```python
from build123d import *

# Parameters (mm, degrees)
BOSS_EXTRUDE1_DEPTH  = 10
CHAMFER1_SIZE        = 5
CHAMFER2_SIZE        = 2
CHAMFER3_SIZE        = 1
CUT_EXTRUDE1_DEPTH   = 3
M3_CLEARANCE_HOLE1_D = 3.4
CUT_EXTRUDE2_DEPTH   = 3


with BuildPart() as part:
    # Sketch1 → Boss-Extrude1 (new body)
    with BuildSketch(Plane(origin=(0, 0, 0), x_dir=(1, 0, 0), z_dir=(0, 1, 0))):
        Polygon((-21, 0), (21, 0), (21, -8), (9.21, -8), (9.21, -30.15), (-9.21, -30.15), (-9.21, -8), (-21, -8), align=None)
        with BuildLine():
            Line((-2, -7.343426738), (-2, -17.343426738))
            ThreePointArc((-2, -17.343426738), (0, -25.45), (2, -17.343426738))
            Line((2, -17.343426738), (2, -7.343426738))
            ThreePointArc((2, -7.343426738), (0, -5.343426738), (-2, -7.343426738))
        make_face(mode=Mode.SUBTRACT)
    extrude(amount=BOSS_EXTRUDE1_DEPTH)

    # Chamfer1
    chamfer1_edges = [part.edges().sort_by_distance(p)[0] for p in [
        (9.21, 5, 30.15),
        (-9.21, 5, 30.15),
    ]]
    chamfer(chamfer1_edges, length=CHAMFER1_SIZE)

    # Chamfer2
    chamfer2_edges = [part.edges().sort_by_distance(p)[0] for p in [
        (-21, 0, 4),
        (21, 10, 4),
        (-21, 10, 4),
        (21, 0, 4),
    ]]
    chamfer(chamfer2_edges, length=CHAMFER2_SIZE)

    # Chamfer3
    chamfer3_edges = [part.edges().sort_by_distance(p)[0] for p in [
        (0, 0, 5.343426738),
        (-2, 0, 12.343426738),
        (0, 0, 25.45),
        (2, 0, 12.343426738),
        (0, 10, 5.343426738),
        (-2, 10, 12.343426738),
        (0, 10, 25.45),
        (2, 10, 12.343426738),
        (0, 0, 0),
        (0, 10, 0),
    ]]
    chamfer(chamfer3_edges, length=CHAMFER3_SIZE)

    # Sketch2 → Cut-Extrude1 (cut)
    with BuildSketch(Plane(origin=(9.21, 0, 0), x_dir=(0, 0, -1), z_dir=(1, 0, 0))):
        Polygon((-10.582508417, 1.95), (-8.821590096, 5), (-10.582508417, 8.05), (-14.104345059, 8.05), (-15.86526338, 5), (-14.104345059, 1.95), align=None)
    extrude(amount=-CUT_EXTRUDE1_DEPTH, mode=Mode.SUBTRACT)

    # Sketch6 → CBORE for M3 Hex Socket Head Cap Screw1 (revolve, cut)
    with BuildSketch(Plane(origin=(-9.21, 5, 12.343426738), x_dir=(0, 0, 1), z_dir=(0, 1, 0))):
        Polygon((0, 0), (0, 30.21), (1.7, 30.21), (1.7, 3.4), (3.25, 3.4), (3.25, 0.025), (3.275, 0), align=None)
    revolve(axis=Axis((-15.56, 5, 12.343426738), (1, 0, 0)), mode=Mode.SUBTRACT)

    # M3 Clearance Hole1 (through all)
    with Locations(Plane(origin=(0, 0, 0), x_dir=(-1, 0, 0), z_dir=(0, 0, -1))):
        with Locations((16, 5), (-16, 5)):
            Hole(M3_CLEARANCE_HOLE1_D / 2)

    # Sketch9 → Cut-Extrude2 (cut)
    with BuildSketch(Plane(origin=(0, 0, 8), x_dir=(-1, 0, 0), z_dir=(0, 0, -1))):
        Polygon((17.760918321, 1.95), (19.521836642, 5), (17.760918321, 8.05), (14.239081679, 8.05), (12.478163358, 5), (14.239081679, 1.95), align=None)
        Polygon((-14.239081679, 1.95), (-17.760918321, 1.95), (-19.521836642, 5), (-17.760918321, 8.05), (-14.239081679, 8.05), (-12.478163358, 5), align=None)
    extrude(amount=CUT_EXTRUDE2_DEPTH, mode=Mode.SUBTRACT)


solid = part.part
```
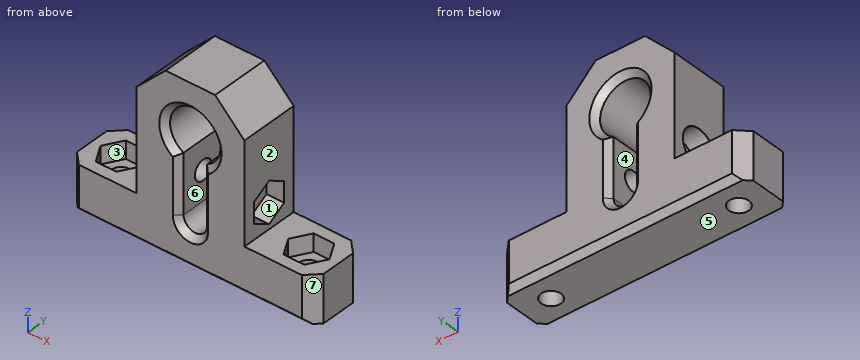
Part model, mm, in its own coordinate system. Face numbers are marked on the shaded views. A direction names the side the tool comes from. Round coordinates to 2 decimals unless told otherwise and drop trailing zeros. Write each loop counter-clockwise with the first axis right and the second up, starting at its lowest first coordinate (ties: lowest second). Pieces come first, ordered by that corner, then holes. Notation, with made-up numbers: (81.5, -38) -> (90.5, -38) arc R18 ccw to (90.5, -16) -> close; hole circle Ø3 at (1, 65). An arc over 180 degrees is marked (long way). Return JSON: item names as keys, results as strings. Group by question number.
Q1. Which spindle directions (+Z, -Z, +X, -X, +Y, -Y) get a long thin tool onto all of the face, cutting with end or side? Do the marked faces 1, 2, 3 and 4. Say none if no direction does.
Q2. Saw through at C-C on y = 4.5. State how many separate pieces and enclosed holes the cut face has, plus the area to 3 significant figures.
Q3. Pin check, flat tips, straight feed: pin 1 (5 mm diameter, centred on x = -15, y = 4.5, fed in from +Z); pin 2 (5 mm diameter, centred on x = 0, z = 21.15, fed in from +Y); pin 3 (1.8 mm diameter, centred on x = 14.5, y = 4.5, fed in from +Z); pin 4 (4.5 mm diameter, centred on y = 5, z = 12.34, fed in from +X). Stop position of each tip, or through.
Q4. Probe L1, parallel to X at y = 5.5, z = 21.15; L2, parallel to Z at x = 11, y = 6.25; L3, parallel to Y at x = 16, z = 2.8. List the from-to ranges inside material, lowest first. Write a range as [from, to].
Q5. Saw through at D-D on x = 16. Write the cut outline in (y, z), plus the area to 3 significant figures.
Q6. Saw through at A-A on x = 7.5. Write the cut outline in (y, z).
Q7. Mould opens along X. For the marked faces 5, 6 and 7 say: pulls with the +X half, pulls with the -X half, needs draft (parallel to the pull), parting line crosses it, or undercut.
Q8. Saw through at B-B on x = 0. Write the cut outline in (y, z).
Answer:
{
 "1": {"face 1": "+X", "face 2": "+Z, +X, +Y, -Y", "face 3": "+Z", "face 4": "+Y, -Y"},
 "2": {"separate pieces": "4", "enclosed holes": "0", "area": "477 mm2"},
 "3": {"pin 1": "z = 8", "pin 2": "through", "pin 3": "z = 5", "pin 4": "x = 6.21"},
 "4": {"L1": "[-9.21, -4.3], [4.3, 9.21]", "L2": "[0, 8]", "L3": "[0, 3.3], [6.7, 10]"},
 "5": {"outline": "(0, 1) -> (1, 0) -> (3.3, 0) -> (3.3, 5) -> (1.95, 5) -> (1.95, 8) -> (0, 8) -> close; (6.7, 0) -> (9, 0) -> (10, 1) -> (10, 8) -> (8.05, 8) -> (8.05, 5) -> (6.7, 5) -> close", "area": "43.7 mm2"},
 "6": {"outline": "(0, 1) -> (1, 0) -> (9, 0) -> (10, 1) -> (10, 26.86) -> (0, 26.86) -> close; hole (1.95, 10.58) -> (5, 8.82) -> (8.05, 10.58) -> (8.05, 14.1) -> (5, 15.87) -> (1.95, 14.1) -> close"},
 "7": {"face 5": "needs draft", "face 6": "undercut", "face 7": "pulls with the +X half"},
 "8": {"outline": "(0, 1) -> (1, 0) -> (9, 0) -> (10, 1) -> (10, 4.34) -> (9, 5.34) -> (1, 5.34) -> (0, 4.34) -> close; (0, 26.45) -> (1, 25.45) -> (9, 25.45) -> (10, 26.45) -> (10, 30.15) -> (0, 30.15) -> close"}
}
